```python
from build123d import *
from OCP.BRepFilletAPI import BRepFilletAPI_MakeChamfer

# Parameters (mm, degrees)
BOSS_EXTRU_1_DEPTH      = 15
CHANFREIN1_SIZE         = 10.503113073
CHANFREIN1_SIZE_2       = 15
ESQUISSE4_R             = 2
ENL_V_MAT_EXTRU_3_DEPTH = 4
ENL_V_MAT_EXTRU_5_DEPTH = 5
ESQUISSE6_R             = 2
ENL_V_MAT_EXTRU_6_DEPTH = 5


with BuildPart() as part:
    # Esquisse1 → Boss.-Extru.1 (new body)
    with BuildSketch(Plane(origin=(0, 0, 0), x_dir=(1, 0, 0), z_dir=(0, 1, 0))):
        Polygon((-41.352348911, -18.647651089), (8.647651089, -18.647651089), (8.647651089, -68.647651089), (68.647651089, -68.647651089), (68.647651089, -46.647651089), (30.647651089, -46.647651089), (30.647651089, 3.352348911), (-19.352348911, 3.352348911), (-19.352348911, 41.352348911), (-19.352348911, 90.352348911), (-41.352348911, 90.352348911), (-41.352348911, 41.352348911), align=None)
    extrude(amount=BOSS_EXTRU_1_DEPTH)

    # Chanfrein1
    chanfrein1_edges_1 = [part.edges().sort_by_distance(p)[0] for p in [
        (38.647651089, 15, 68.647651089),
    ]]
    chanfrein1_side_1 = [part.faces().sort_by_distance(p)[0] for p in [
        (38.647651089, 15, 68.437588827),
    ]]
    chanfrein1_edges_2 = [part.edges().sort_by_distance(p)[0] for p in [
        (8.647651089, 15, 43.647651089),
    ]]
    chanfrein1_side_2 = [part.faces().sort_by_distance(p)[0] for p in [
        (8.85771335, 15, 43.647651089),
    ]]
    chanfrein1_edges_3 = [part.edges().sort_by_distance(p)[0] for p in [
        (-16.352348911, 15, 18.647651089),
    ]]
    chanfrein1_side_3 = [part.faces().sort_by_distance(p)[0] for p in [
        (-16.352348911, 14.789937739, 18.647651089),
    ]]
    chanfrein1_edges_4 = [part.edges().sort_by_distance(p)[0] for p in [
        (-41.352348911, 15, -35.852348911),
    ]]
    chanfrein1_side_4 = [part.faces().sort_by_distance(p)[0] for p in [
        (-41.14228665, 15, -35.852348911),
    ]]
    chanfrein1 = BRepFilletAPI_MakeChamfer(part.part.solid().wrapped)
    for e in chanfrein1_edges_1:
        chanfrein1.Add(CHANFREIN1_SIZE - 0.0001, CHANFREIN1_SIZE_2 - 0.0001, e.wrapped, chanfrein1_side_1[0].wrapped)
    for e in chanfrein1_edges_2:
        chanfrein1.Add(CHANFREIN1_SIZE - 0.0001, CHANFREIN1_SIZE_2 - 0.0001, e.wrapped, chanfrein1_side_2[0].wrapped)
    for e in chanfrein1_edges_3:
        chanfrein1.Add(CHANFREIN1_SIZE_2 - 0.0001, CHANFREIN1_SIZE - 0.0001, e.wrapped, chanfrein1_side_3[0].wrapped)
    for e in chanfrein1_edges_4:
        chanfrein1.Add(CHANFREIN1_SIZE - 0.0001, CHANFREIN1_SIZE_2 - 0.0001, e.wrapped, chanfrein1_side_4[0].wrapped)
    add(Compound.cast(chanfrein1.Shape()), mode=Mode.REPLACE)  # a hair under: the kernel refuses the full size

    # Esquisse4 → Enlèv. mat.-Extru.3 (cut)
    with BuildSketch(Plane.XZ):
        with Locations(Location((38.647651089, 63.647651089, 0), (0, 0, 270))):
            Circle(ESQUISSE4_R)
        with Locations(Location((13.647651089, 38.647651089, 0), (0, 0, 270))):
            Circle(ESQUISSE4_R)
        with Locations(Location((-11.352348911, 13.647651089, 0), (0, 0, 270))):
            Circle(ESQUISSE4_R)
    extrude(amount=-ENL_V_MAT_EXTRU_3_DEPTH, mode=Mode.SUBTRACT)

    # Esquisse5 → Enlèv. mat.-Extru.5 (cut)
    with BuildSketch(Plane(origin=(0, 15, 0), x_dir=(1, 0, 0), z_dir=(0, 1, 0))):
        Polygon((-19.352348911, 3.352348911), (30.647651089, 3.352348911), (30.647651089, -46.647651089), (68.647651089, -46.647651089), (68.647651089, -56.140382231), (21.150764162, -56.140382231), (21.150764162, -6.144538016), (-28.849235838, -6.144538016), (-28.849235838, 90.352348911), (-19.352348911, 90.352348911), align=None)
    extrude(amount=-ENL_V_MAT_EXTRU_5_DEPTH, mode=Mode.SUBTRACT)

    # Esquisse6 → Enlèv. mat.-Extru.6 (cut)
    with BuildSketch(Plane(origin=(0, 10, 0), x_dir=(1, 0, 0), z_dir=(0, 1, 0))):
        with Locations(Location((-23.849235838, 78.855461984, 0), (0, 0, 270))):
            Circle(ESQUISSE6_R)
        with Locations(Location((26.150764162, -1.144538016, 0), (0, 0, 270))):
            Circle(ESQUISSE6_R)
        with Locations(Location((56.150764162, -51.140382231, 0), (0, 0, 270))):
            Circle(ESQUISSE6_R)
    extrude(amount=-ENL_V_MAT_EXTRU_6_DEPTH, mode=Mode.SUBTRACT)


solid = part.part
```
Geometry check sheet. Reference: the model listing, model coordinates, mm. A direction names the side the tool comes from. Round coordinates to 2 decimals unless told otherwise and drop trailing zeros. Order: outer loops, then holes, each group sorted by start corner. A loop starts at its lowest first (then second) coordinate and runs counter-clockwise, first axis right, second up. Notation, with made-up numbers: (40.5, -5.75) -> (96.5, -5.75) arc R17 cw to (96.5, 16.25) -> close; hole circle Ø6 at (-25.75, 79). An arc over 180 degrees is marked (long way). Return JSON: item names as keys, results as strings. Group by question number.
Q1. Material ranges on probe 1 along Z at (x, y) = (-25.5, 5.25); probe 2 along Y at (x, z) = (38, 56); probe 3 along X at (y, z) = (1.25, 37.5), recorded low to high. Write a range as from..to.
Q2. Gauge pin test, flat ends, axial feed: pin 1 (2.5 mm diameter, centred on x = 0, y = 12, fed in from -Z); pin 2 (5 mm diameter, centred on x = 4.5, y = 7.5, fed in from -Z); pin 3 (3.5 mm diameter, centred on x = -11.35, z = 13.65, fed in from +Y); pin 4 (10 mm diameter, centred on x = 4, z = -12, fed in from +Y). Record the tip position at first contact, or that the pin passes through.
Q3. Tool access check on faces 1 (the cylindrical face through (40.334, 1.972, 62.572)), 2 (the flat face through (45, 13, 56.14)), 3 (the flat face through (26, 5, 1)), 4 (the flat face through (-19.352, 5, -46)), 5 (the flat face through (-11.52, 7.61, 13.32)). Record the directions out of +Z, -Z, +X, -X, +Y, -Y that give a thin tool (end or side, any length) a straight path to the whole face; none if there is none.
Q4. Section check B-B, the plane y = 7.5. Record the boundary of the cut face in (x, z), plus the area to 3 significant figures.
Numbers:
{
 "1": {"probe 1": "-90.35..-79.98, -77.73..14.97", "probe 2": "0..10", "probe 3": "9.52..12.01, 15.29..30.65"},
 "2": {"pin 1": "z = 6.14", "pin 2": "z = -3.35", "pin 3": "y = 9.64", "pin 4": "through"},
 "3": {"face 1": "-Y", "face 2": "-Z, +X, +Y", "face 3": "+Y", "face 4": "-Z, +X, +Y, -Y", "face 5": "+Z, -X, +Y"},
 "4": {"outline": "(-36.1, -90.35) -> (-19.35, -90.35) -> (-19.35, -3.35) -> (30.65, -3.35) -> (30.65, 46.65) -> (68.65, 46.65) -> (68.65, 63.4) -> (13.9, 63.4) -> (13.9, 13.4) -> (-36.1, 13.4) -> close; hole circle Ø4 at (-23.85, -78.86); hole circle Ø4 at (26.15, 1.14); hole circle Ø4 at (56.15, 51.14)", "area": "4,010 mm^2"}
}
